```python
from build123d import *

# Parameters (mm, degrees)
SKETCH1_W               = 38.1
SKETCH1_H               = 30.48
BOSS_EXTRUDE1_DEPTH     = 2.54
SKETCH2_R               = 0.8509
CUT_EXTRUDE1_DEPTH      = 2.54
MIRROR2_COPY_1_SKETCH_R = 0.8509
MIRROR2_COPY_1_DEPTH    = 2.54
FILLET1_R               = 6.35
SKETCH3_W               = 15.24
SKETCH3_H               = 4.7752
CUT_EXTRUDE2_DEPTH      = 2.54


with BuildPart() as part:
    # Sketch1 → Boss-Extrude1 (new body)
    with BuildSketch(Plane(origin=(0, 0, 0), x_dir=(0, 0, -1), z_dir=(1, 0, 0))):
        Rectangle(SKETCH1_W, SKETCH1_H)
    extrude(amount=BOSS_EXTRUDE1_DEPTH)

    # Sketch2 → Cut-Extrude1 (cut)
    with BuildSketch(Plane(origin=(2.54, 0, 0), x_dir=(0, 0, -1), z_dir=(1, 0, 0))):
        with Locations((10.16, 6.35)):
            Circle(SKETCH2_R)
    cut_extrude1 = extrude(amount=-CUT_EXTRUDE1_DEPTH, mode=Mode.SUBTRACT)

    # Mirror1: Cut-Extrude1 across plane
    add(cut_extrude1.mirror(Plane.XY), mode=Mode.SUBTRACT)

    # Mirror2: Cut-Extrude1 across plane
    add(cut_extrude1.mirror(Plane.ZX), mode=Mode.SUBTRACT)

    # Mirror2 copy 1 sketch → Mirror2 copy 1 (cut)
    with BuildSketch(Plane(origin=(2.54, 0, 0), x_dir=(0, 0, 1), z_dir=(1, 0, 0))):
        with Locations((10.16, 6.35)):
            Circle(MIRROR2_COPY_1_SKETCH_R)
    extrude(amount=-MIRROR2_COPY_1_DEPTH, mode=Mode.SUBTRACT)

    # Fillet1
    fillet1_edges = [part.edges().sort_by_distance(p)[0] for p in [
        (1.27, -15.24, -19.05),
        (1.27, -15.24, 19.05),
        (1.27, 15.24, 19.05),
        (1.27, 15.24, -19.05),
    ]]
    fillet(fillet1_edges, radius=FILLET1_R)

    # Sketch3 → Cut-Extrude2 (cut)
    with BuildSketch(Plane(origin=(2.54, 0, 0), x_dir=(0, 0, -1), z_dir=(1, 0, 0))):
        with Locations((0, -6.35)):
            Rectangle(SKETCH3_W, SKETCH3_H)
    extrude(amount=-CUT_EXTRUDE2_DEPTH, mode=Mode.SUBTRACT)


solid = part.part
```
Verification items for the finished model (mm, model axes). A direction names the side the tool comes from. Coordinates: 2 decimals unless noted, no trailing zeros. Write each loop counter-clockwise with the first axis right and the second up, starting at its lowest first coordinate (ties: lowest second). Pieces come first, ordered by that corner, then holes. Notation, with made-up numbers: (60.25, -18) - (66.25, -18) arc R25 ccw to (66.25, 16) - close; hole circle Ø10 at (3, 87). An arc over 180 degrees is marked (long way). Write item = value, one per line.
Q1. Access from +Z, -Z, +X, -X, +Y, -Y to the whole of each face (thin tool, end or side, straight path). Record for faces 4 (the face through (1, -3.962, 0)), 5 (the face through (1.29, 13.43, -17.14)).
Answer:
face_4 = +X, -X
face_5 = -Z, +X, -X, +Y
Q2. Cross-section at B-B (z = -10.16). Enter the section's corners in (x, y), plus the area to 3 significant figures.
Answer:
outline = (0, -15.24) - (2.54, -15.24) - (2.54, -7.2) - (0, -7.2) - close; (0, -5.5) - (2.54, -5.5) - (2.54, 5.5) - (0, 5.5) - close; (0, 7.2) - (2.54, 7.2) - (2.54, 15.24) - (0, 15.24) - close
area = 68.8 mm²
Q3. Material ranges on L1, parallel to Y at x = 1.3, z = -10.16; L2, parallel to Z at x = 0.75, y = -6.35; L3, parallel to Y at x = 1.15, z = -6, recorded low to high. Write a range as from..to.
Answer:
L1 = -15.24..-7.2, -5.5..5.5, 7.2..15.24
L2 = -19.05..-11.01, -9.31..-7.62, 7.62..9.31, 11.01..19.05
L3 = -15.24..-8.74, -3.96..15.24
Q4. Cross-section at A-A (y = -6.35). Enter the section's corners in (x, z).
Answer:
outline = (0, -19.05) - (2.54, -19.05) - (2.54, -11.01) - (0, -11.01) - close; (0, -9.31) - (2.54, -9.31) - (2.54, -7.62) - (0, -7.62) - close; (0, 7.62) - (2.54, 7.62) - (2.54, 9.31) - (0, 9.31) - close; (0, 11.01) - (2.54, 11.01) - (2.54, 19.05) - (0, 19.05) - close
Q5. Mould release check, pull along Z, two halves, no side actions. Record for faces 1 (the face through (2.54, 0, 0)), 2 (the face through (1.29, -13.33, 17.24)), 3 (the face through (1.29, 6.39, 9.31)): released by +Z, released by -Z, zero draft, split by the parting line, or undercut.
Answer:
face_1 = zero draft
face_2 = released by +Z
face_3 = undercut
Q6. Cross-section at D-D (z = 16.5). Enter the section's corners in (x, y), plus the area to 3 significant figures.
Answer:
outline = (0, -13.98) - (2.54, -13.98) - (2.54, 13.98) - (0, 13.98) - close
area = 71.0 mm²
Q7. Cross-section at C-C (x = 1.25). Enter the section's corners in (y, z), plus the area to 3 significant figures.
Answer:
outline = (-15.24, -12.7) arc R6.35 ccw to (-8.89, -19.05) - (8.89, -19.05) arc R6.35 ccw to (15.24, -12.7) - (15.24, 12.7) arc R6.35 ccw to (8.89, 19.05) - (-8.89, 19.05) arc R6.35 ccw to (-15.24, 12.7) - close; hole (-8.74, -7.62) - (-3.96, -7.62) - (-3.96, 7.62) - (-8.74, 7.62) - close; hole circle Ø1.7 at (-6.35, -10.16); hole circle Ø1.7 at (-6.35, 10.16); hole circle Ø1.7 at (6.35, -10.16); hole circle Ø1.7 at (6.35, 10.16)
area = 1,040 mm²
Q8. Go/stop test with flat-tipped pins: pin 1 Ø1.4 at (y, z) = (-6.35, 10.16) entering from +X; pin 2 Ø10 at (y, z) = (-2.5, 8) entering from -X. Record where each tip stops, or that it passes through.
Answer:
pin_1 = through
pin_2 = 0
